```python
from build123d import *

# Parameters (mm, degrees)
F0_R     = 55.8162031388
F0_R_2   = 53.34
F1_DEPTH = 25.4
F2_DEPTH = 5.08
F3_W     = 13.5487690568
F3_H     = 3.1119100749
F3_W_2   = 8.3945244551
F3_H_2   = 4.1670650244
F3_W_3   = 7.9046934843
F3_H_3   = 4.2887181044
F3_W_4   = 5.7976543903
F3_H_4   = 3.6839321256
F3_W_5   = 8.4092468023
F3_H_5   = 3.7000700831
F3_W_6   = 10.0910961628
F3_H_6   = 4.372805357
F3_W_7   = 8.8297128677
F3_H_7   = 4.6250857413
F3_W_8   = 6.8733096123
F3_H_8   = 3.6097243428
F3_W_9   = 6.8847164512
F3_H_9   = 3.6839284003
F3_W_10  = 7.9117268324
F3_H_10  = 4.2525529861
F3_W_11  = 10.2453604341
F3_H_11  = 3.1119063497
F3_W_12  = 9.3357227743
F3_H_12  = 3.9257928729
F3_W_13  = 9.9581070244
F3_H_13  = 4.0215402842
F3_W_14  = 13.9796473086
F3_H_14  = 3.9736665785
F3_W_15  = 11.2507455051
F3_H_15  = 3.8300380111
F3_W_16  = 11.3943703473
F3_H_16  = 3.3991634846
F3_W_17  = 7.6600834727
F3_H_17  = 3.5427883267
F3_W_18  = 9.4169080257
F3_H_18  = 3.7821643054
F3_W_19  = 9.1442242265
F3_H_19  = 3.8300417364
F3_W_20  = 10.7719898224
F3_W_21  = 5.6493058801
F3_H_20  = 12.7348862588
F3_W_22  = 2.7767792344
F3_H_21  = 12.112505734
F3_W_23  = 5.8886855841
F3_H_22  = 12.7827599645
F3_W_24  = 12.351885438
F3_H_23  = 6.3195675611
F3_W_25  = 5.2663087845
F3_H_24  = 3.6385394633
F3_W_26  = 3.6878287792
F3_H_25  = 15.8802717924
F3_W_27  = 5.7199150324
F3_H_26  = 17.6865570247
F3_W_28  = 4.3651908636
F3_H_27  = 14.2245069146
F3_W_29  = 59.7025379539
F3_H_28  = 2.6341676712
F3_W_30  = 102.2809818387
F3_H_29  = 3.7544369698
F3_W_31  = 101.4531031251
F3_H_30  = 4.5157186687
F3_W_32  = 50.049200654
F3_H_31  = 3.6878362298
F3_W_33  = 70.2946484089
F3_H_32  = 3.7630945444
F3_W_34  = 87.4543711543
F3_H_33  = 4.1394084692
F3_W_35  = 94.1526964307
F3_H_34  = 4.5157149434
F4_DEPTH = 25.4


# Not quite as in the source:
# - a fillet or chamfer that OpenCascade refuses, or shapes differently, is made with other operations: its cross-section is extruded or revolved along the edge and cut away or added


with BuildPart() as f1:
    # F0 (on Front) → F1 (new body)
    with BuildSketch(Plane.XZ):
        Circle(F0_R)
        Circle(F0_R_2, mode=Mode.SUBTRACT)
    extrude(amount=-F1_DEPTH)

    # F0 (on Front) → F2 (join)
    with BuildSketch(Plane.XZ):
        Circle(F0_R_2)
    extrude(amount=-F2_DEPTH)

    # F3 (on face) → F4 (cut)
    with BuildSketch(Plane.XZ):
        with Locations((1.637134701, 50.0085186213)):
            Rectangle(F3_W, F3_H)
        with Locations((1.3199597597, 44.4235429168)):
            Rectangle(F3_W_2, F3_H_2)
        with Locations((-11.756375432, 44.2828312516)):
            Rectangle(F3_W_3, F3_H_3)
        with Locations((-24.4977399707, 43.2760901749)):
            Rectangle(F3_W_4, F3_H_4)
        with Locations((-30.0885364413, 36.9247384369)):
            Rectangle(F3_W_5, F3_H_5)
        with Locations((-17.0542001724, 36.4201851189)):
            Rectangle(F3_W_6, F3_H_6)
        with Locations((0.1427084208, 37.387246266)):
            Rectangle(F3_W_7, F3_H_7)
        with Locations((13.7023478746, 36.8178598583)):
            Rectangle(F3_W_8, F3_H_8)
        with Locations((15.9046910703, 44.2423652858)):
            Rectangle(F3_W_9, F3_H_9)
        with Locations((27.7209356427, 36.6447903216)):
            Rectangle(F3_W_10, F3_H_10)
        with Locations((-21.367046982, 30.954066664)):
            Rectangle(F3_W_11, F3_H_11)
        with Locations((-35.5621371418, 28.5363532603)):
            Rectangle(F3_W_12, F3_H_12)
        with Locations((-24.3832040578, 24.2754332721)):
            Rectangle(F3_W_13, F3_H_13)
        with Locations((-25.7237199694, 15.490276739)):
            Rectangle(F3_W_14, F3_H_14)
        with Locations((-38.0516629666, 20.3017666936)):
            Rectangle(F3_W_15, F3_H_15)
        with Locations((-44.5387940854, 14.9157717824)):
            Rectangle(F3_W_16, F3_H_16)
        with Locations((-7.6746530831, 30.0683714449)):
            Rectangle(F3_W_17, F3_H_17)
        with Locations((4.7084540129, 30.4753128439)):
            Rectangle(F3_W_18, F3_H_18)
        with Locations((18.1541852653, 29.8289936036)):
            Rectangle(F3_W_19, F3_H_19)
        with Locations((33.2828462124, 29.7093037516)):
            Rectangle(F3_W_20, F3_H_18)
        with Locations((-12.0791979134, 19.6315106004)):
            Rectangle(F3_W_21, F3_H_20)
        with Locations((-5.5681280792, 18.8894383609)):
            Rectangle(F3_W_22, F3_H_21)
        with Locations((1.3020038605, 18.7458135188)):
            Rectangle(F3_W_23, F3_H_22)
        with Locations((13.1990686059, 21.9295322895)):
            Rectangle(F3_W_24, F3_H_23)
        with Locations((13.1033211946, 13.8385724276)):
            Rectangle(F3_W_25, F3_H_24)
        with Locations((23.8093435764, 17.1886943281)):
            Rectangle(F3_W_26, F3_H_25)
        with Locations((34.458912909, 15.457669273)):
            Rectangle(F3_W_27, F3_H_26)
        with Locations((44.544018805, 14.2534784973)):
            Rectangle(F3_W_28, F3_H_27)
        with Locations((-19.3811021745, 7.7809505165)):
            Rectangle(F3_W_29, F3_H_28)
        with Locations((0.4028789699, 1.8772184849)):
            Rectangle(F3_W_30, F3_H_29)
        with Locations((0.5910359323, -7.5348559767)):
            Rectangle(F3_W_31, F3_H_30)
        with Locations((0.026576221, -44.526103884)):
            Rectangle(F3_W_32, F3_H_31)
        with Locations((-0.3873705864, -35.0054651499)):
            Rectangle(F3_W_33, F3_H_32)
        with Locations((0.1394636929, -25.7858783007)):
            Rectangle(F3_W_34, F3_H_33)
        with Locations((0.4781447351, -16.8673358858)):
            Rectangle(F3_W_35, F3_H_34)
    extrude(amount=-F4_DEPTH, mode=Mode.SUBTRACT)

    # F5: fillet of radius 2.54 on 2 edges, made by hand

    # F5_s1 → F5_t2 (revolve, cut)
    with BuildSketch(Plane.XY):
        with BuildLine():
            ThreePointArc((55.8162031388, 2.54), (55.072254363, 0.7439487758), (53.2762031388, 0))
            Line((53.2762031388, 0), (55.8162031388, 0))
            Line((55.8162031388, 0), (55.8162031388, 2.54))
        make_face()
    revolve(axis=Axis((0, 0, 0), (0, -1, 0)), mode=Mode.SUBTRACT)

    # F5_s3 → F5_t4 (revolve, cut)
    with BuildSketch(Plane.XY):
        with BuildLine():
            ThreePointArc((55.88, 25.4), (54.0839487758, 24.6560512242), (53.34, 22.86))
            Line((53.34, 22.86), (53.34, 25.4))
            Line((53.34, 25.4), (55.88, 25.4))
        make_face()
    revolve(axis=Axis((0, 25.4, 0), (0, -1, 0)), mode=Mode.SUBTRACT)


solid = f1.part
```
Can you work these out from the model? Positions are in its coordinate system, mm. Coordinates: 2 decimals unless noted, no trailing zeros. Loops run counter-clockwise (first coordinate to the right, second up) from the corner with the lowest first, then second, coordinate; pieces in that order, holes last.
Item 1: Please list where these lines run through material, in increasing order: L1, parallel to Z at x = 0, y = 11.5; L2, parallel to Y at x = 19.5, z = 4.5; L3, parallel to Z at x = 4, y = 7.5.
Answers below:
L1: z = -55.82 to -53.34, 53.34 to 55.82
L2: y = 0 to 5.08
L3: z = -55.67 to -53.19, 53.19 to 55.67
Item 2: Suppose I cut it at B-B (x = -45). State how many separate pieces and enclosed holes the cut face has, then the cut area to 3 significant figures.
Answers below:
separate pieces: 6
enclosed holes: 0
area: 408 mm2
Item 3: I'm going to push flat-ended pins straight in: pin 1 (4 mm diameter, centred on y = 3.5, z = 37.5, fed in from -X); pin 2 (10 mm diameter, centred on x = -16, y = 14, fed in from -Z); pin 3 (4 mm diameter, centred on y = 19, z = 40.5, fed in from +X); pin 4 (1 mm diameter, centred on x = 17, z = -17.5, fed in from -Y). Where does each tip first touch, or does it pass through?
Answers below:
pin 1: stops at x = -43.07
pin 2: stops at z = -54.72
pin 3: stops at x = 40.41
pin 4: passes through
Item 4: Suppose I cut it at A-A (y = 20.75). Please give me the cut outline in (x, z), then the cut area to 3 significant figures.
Answers below:
outline: circle Ø111.63 at (0, 0); hole circle Ø106.68 at (0, 0)
area: 849 mm2
